Autodesk Inventor part; units mm, degrees
ref_plane "or_XY" through (0, 0, 0) normal (0, 0, 1) x (1, 0, 0)
ref_plane "or_YZ" through (0, 0, 0) normal (1, 0, 0) x (0, 1, 0)
ref_plane "or_ZX" through (0, 0, 0) normal (0, 1, 0) x (0, 0, 1)
sketch "Sketch_9" plane through (0, 0, 0) normal (0, 0, 1) x (1, 0, 0)
  line L0 (50, 0) -> (-50, 0)
  line L1 (0, 4.85) -> (0, 4.2)
  line L2 (0, 4.2) -> (0.075, 4.2)
  arc A0 (0.225, 4.05) -> (0.075, 4.2) centre (0.075, 4.05) ccw
  line L3 (0.225, 4.05) -> (0.225, 3.9)
  line L4 (0.225, 3.9) -> (1.6031, 3.9)
  arc A1 (2.3969, 3.9) -> (1.6031, 3.9) centre (2, 3.45) ccw
  line L5 (2.3969, 3.9) -> (3.775, 3.9)
  line L6 (3.775, 3.9) -> (3.775, 4.05)
  arc A2 (3.925, 4.2) -> (3.775, 4.05) centre (3.925, 4.05) ccw
  line L7 (3.925, 4.2) -> (4, 4.2)
  line L8 (4, 4.2) -> (4, 4.85)
  arc A3 (4, 4.85) -> (3.85, 5) centre (3.85, 4.85) ccw
  line L9 (3.85, 5) -> (0.15, 5)
  arc A4 (0.15, 5) -> (0, 4.85) centre (0.15, 4.85) ccw
revolve "Revolution1" add sketch "Sketch_9" angle 360 about axis through (50, 0, 0) along (1, 0, 0)
ref_plane "or_XY" through (0, 0, 0) normal (0, 0, 1) x (1, 0, 0)
ref_plane "or_YZ" through (0, 0, 0) normal (1, 0, 0) x (0, 1, 0)
ref_plane "or_ZX" through (0, 0, 0) normal (0, 1, 0) x (0, 0, 1)
properties part number "SKF_WBB1-8705-2RS1_or"
Read the model definition and answer for the solid it produces. Units are mm, in the model's axes. Round coordinates to 2 decimals unless told otherwise and drop trailing zeros. Loops run counter-clockwise (first coordinate to the right, second up) from the corner with the lowest first, then second, coordinate; pieces in that order, holes last.
Q1. Determine the mould class of faces 1 (the face through (1.97, -1.08, 4.88)), 2 (the face through (0.92, -2.87, 2.64)), 3 (the face through (4, -4, 2)) for opening direction Z: released by +Z, released by -Z, zero draft, split by the parting line, or undercut.
Q2. Section C-C on x = 0.4 is taken. Write down the section's boundary in (y, z).
Q3. Consider probe 1 along Z at (x, y) = (1.15, 0); probe 2 along Y at (x, z) = (3.6, 1.5); probe 3 along Y at (x, z) = (2.9, 2). Determine where each line is inside the solid, lowest interval first.
Q4. Section A-A on z = 0 is taken. Write down the section's boundary in (x, y) (3 decimals), and give its area (3 significant figures).
Q5. Each of these flat-tipped pins is pushed along its axis until it touches: pin 1 (1.5 mm diameter, centred on x = 0.5, y = 2.5, fed in from -Z); pin 2 (2.5 mm diameter, centred on y = -1.5, z = 0.5, fed in from +X); pin 3 (2 mm diameter, centred on x = 0.5, y = -1.5, fed in from +Z). Where does it stop, or does it pass through?
Output:
1. face 1: split by the parting line
1. face 2: undercut
1. face 3: zero draft
2. outline: circle Ø10 at (0, 0); hole circle Ø7.8 at (0, 0)
3. probe 1: z = -5 to -3.9, 3.9 to 5
3. probe 2: y = -4.77 to -3.6, 3.6 to 4.77
3. probe 3: y = -4.58 to -3.35, 3.35 to 4.58
4. outline: (0, -4.85) arc R0.15 ccw to (0.15, -5) - (3.85, -5) arc R0.15 ccw to (4, -4.85) - (4, -4.2) - (3.925, -4.2) arc R0.15 cw to (3.775, -4.05) - (3.775, -3.9) - (2.397, -3.9) arc R0.6 cw to (1.603, -3.9) - (0.225, -3.9) - (0.225, -4.05) arc R0.15 cw to (0.075, -4.2) - (0, -4.2) - close; (0, 4.2) - (0.075, 4.2) arc R0.15 cw to (0.225, 4.05) - (0.225, 3.9) - (1.603, 3.9) arc R0.6 cw to (2.397, 3.9) - (3.775, 3.9) - (3.775, 4.05) arc R0.15 cw to (3.925, 4.2) - (4, 4.2) - (4, 4.85) arc R0.15 ccw to (3.85, 5) - (0.15, 5) arc R0.15 ccw to (0, 4.85) - close
4. area: 8.37 mm2
5. pin 1: stops at z = -4.68
5. pin 2: passes through
5. pin 3: stops at z = 4.97
